For this review, take the finished solid that the model builds, in its own axes (mm). A direction names the side the tool comes from. Give positions to 0.01 mm unless a question says otherwise; leave off trailing zeros. Write each loop counter-clockwise with the first axis right and the second up, starting at its lowest first coordinate (ties: lowest second). Pieces come first, ordered by that corner, then holes. Notation, with made-up numbers: M 75,-13.75 L 131,-13.75 A18 ccw 131,14.25 Z; hole C 56.25,-12.5 d3. An arc over 180 degrees is marked long. One line per item, written item: value. Start each with the question number.
Item 1: To check wall thickness, follow probe 1 along Z at (x, y) = (7.5, 12.5); probe 2 along X at (y, z) = (5.75, -11); probe 3 along Z at (x, y) = (32.5, 8.5). State the ranges of each line that lie inside material, in increasing order.
Item 2: Tool access review of faces 1 (the face through (33, 0, -2.6)), 2 (the face through (50, 7, -4)): name each direction out of +Z, -Z, +X, -X, +Y, -Y from which nothing blocks a thin tool from reaching the whole face with its end or side.
Item 3: Consider section C-C, the plane y = 10.5. Write out the cut boundary in (x, z), and give its area (3 significant figures).
Item 4: Consider section D-D, the plane z = -18. Write out the cut boundary in (x, y), and give its area (3 significant figures).
Item 5: Mouldability with a two-part tool opening along Z and no side actions: class faces 3 (the face through (33, 7, 0)), 4 (the face through (61.026, 7.395, -11.481)), 5 (the face through (33, 8, -3)), 6 (the face through (65, 8, -41)) as released by +Z, released by -Z, zero draft, split by the parting line, or undercut.
Item 6: Consider section B-B, the plane x = 59.5. Write out the cut boundary in (y, z).
Item 7: Consider section A-A, the plane z = -11. Write out the cut boundary in (x, y), and give its area (3 significant figures).
Item 8: Clearance check with a flat-ended pin moving along its axis: pin 1 Ø1.9 at (x, z) = (7.5, -31) entering from +Y. State where the tip first meets the part, or that it passes through.
```python
from build123d import *

# Parameters (mm, degrees)
SKETCH1_W           = 67
SKETCH1_H           = 42
SKETCH1_R           = 1.6
BOSS_EXTRUDE1_DEPTH = 15
SKETCH2_W           = 37
SKETCH2_H           = 36
CUT_EXTRUDE1_DEPTH  = 16
FILLET1_R           = 5


with BuildPart() as part:
    # Sketch1 → Boss-Extrude1 (new body)
    with BuildSketch(Plane(origin=(0, 0, 0), x_dir=(1, 0, 0), z_dir=(0, 1, 0))):
        with Locations((33.5, 21)):
            Rectangle(SKETCH1_W, SKETCH1_H)
        with Locations((7.5, 31)):
            Circle(SKETCH1_R, mode=Mode.SUBTRACT)
        with Locations((7.5, 11)):
            Circle(SKETCH1_R, mode=Mode.SUBTRACT)
        with Locations((59.5, 11)):
            Circle(SKETCH1_R, mode=Mode.SUBTRACT)
        with Locations((59.5, 31)):
            Circle(SKETCH1_R, mode=Mode.SUBTRACT)
    extrude(amount=BOSS_EXTRUDE1_DEPTH)

    # Sketch2 → Cut-Extrude1 (cut, through all)
    with BuildSketch(Plane(origin=(0, 15, 0), x_dir=(1, 0, 0), z_dir=(0, 1, 0))):
        with Locations((33.5, 21)):
            Rectangle(SKETCH2_W, SKETCH2_H)
    extrude(amount=-CUT_EXTRUDE1_DEPTH, mode=Mode.SUBTRACT)

    # Fillet1
    fillet1_edges = [part.edges().sort_by_distance(p)[0] for p in [
        (52, 7.5, -39),
        (52, 7.5, -3),
        (15, 7.5, -3),
        (15, 7.5, -39),
        (0, 7.5, -42),
        (67, 7.5, -42),
        (67, 7.5, 0),
        (0, 7.5, 0),
    ]]
    fillet(fillet1_edges, radius=FILLET1_R)


solid = part.part
```
Model answer:
1. probe 1: z = -42 to -32.6, -29.4 to -12.6, -9.4 to 0
1. probe 2: x = 0 to 5.9, 9.1 to 15, 52 to 57.9, 61.1 to 67
1. probe 3: z = -42 to -39, -3 to 0
2. face 1: +Z, -Z, +X, -X, -Y
2. face 2: +Y, -Y
3. outline: M 0,-37 A5 ccw 5,-42 L 62,-42 A5 ccw 67,-37 L 67,-5 A5 ccw 62,0 L 5,0 A5 ccw 0,-5 Z; hole C 7.5,-31 d3.2; hole C 7.5,-11 d3.2; hole M 15,-34 A5 ccw 20,-39 L 47,-39 A5 ccw 52,-34 L 52,-8 A5 ccw 47,-3 L 20,-3 A5 ccw 15,-8 Z; hole C 59.5,-31 d3.2; hole C 59.5,-11 d3.2
3. area: 1,450 mm2
4. outline: M 0,0 L 15,0 L 15,15 L 0,15 Z; M 52,0 L 67,0 L 67,15 L 52,15 Z
4. area: 450 mm2
5. face 3: released by +Z
5. face 4: undercut
5. face 5: undercut
5. face 6: released by -Z
6. outline: M 0,-42 L 15,-42 L 15,-32.6 L 0,-32.6 Z; M 0,-29.4 L 15,-29.4 L 15,-12.6 L 0,-12.6 Z; M 0,-9.4 L 15,-9.4 L 15,0 L 0,0 Z
7. outline: M 0,0 L 5.9,0 L 5.9,15 L 0,15 Z; M 9.1,0 L 15,0 L 15,15 L 9.1,15 Z; M 52,0 L 57.9,0 L 57.9,15 L 52,15 Z; M 61.1,0 L 67,0 L 67,15 L 61.1,15 Z
7. area: 354 mm2
8. pin 1: passes through
